Job drawing, mm, ordinate dimensions from the low corner. One solid piece. A direction names the side the tool comes from. Round coordinates to 2 decimals unless told otherwise and drop trailing zeros. Loops run counter-clockwise (first coordinate to the right, second up) from the corner with the lowest first, then second, coordinate; pieces in that order, holes last. Notation, with made-up numbers: M 17,38.25 L 23,38.25 A22 cw 23,63.25 Z; hole C -16,24.5 d8. An arc over 180 degrees is marked long. One line per item, written item: value.
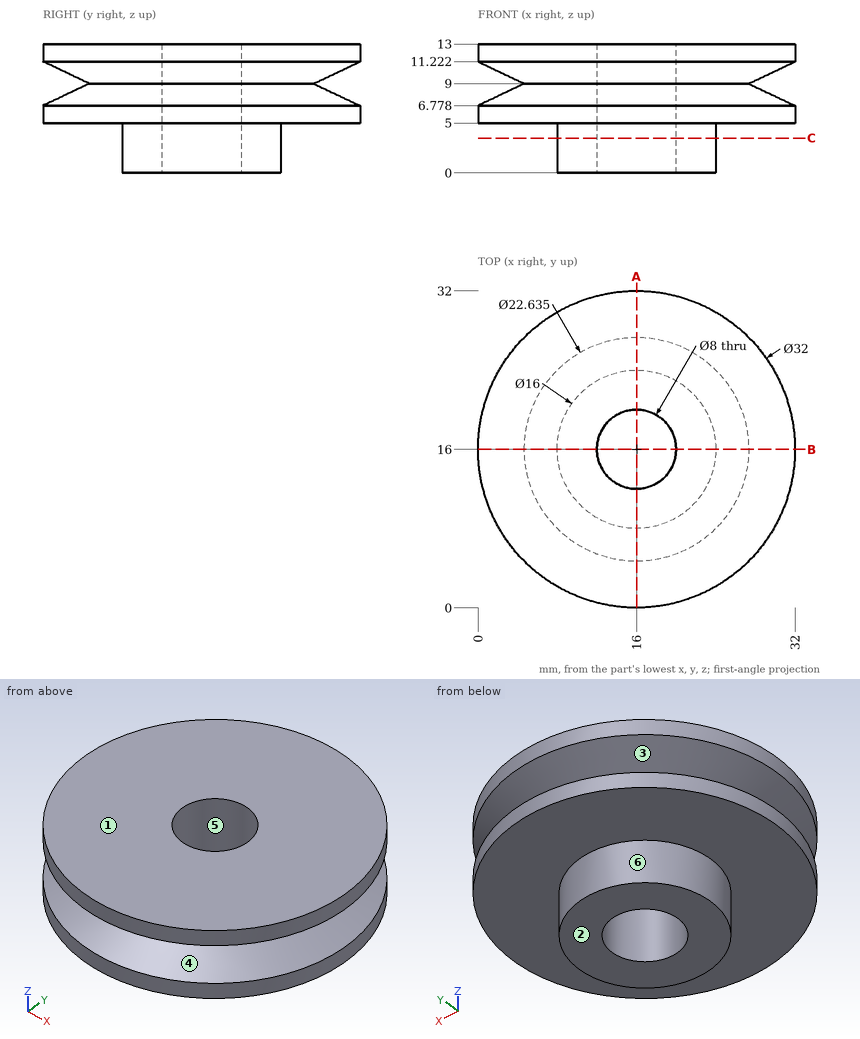
Item 1: Wall check: line 1 along Y through (x, z) = (16, 4); line 2 along Z through (x, y) = (23.5, 10); line 3 along Z through (x, y) = (8.5, 29). Give the ranges that are in metal, low to high.
Check values:
line 1: y = 8 to 12, 20 to 24
line 2: z = 5 to 13
line 3: z = 5 to 7.25, 10.75 to 13
Item 2: Drop flat-ended pins along their axis: P1, Ø2, axis at x = 17, y = 11, coming from the -Z side; P2, Ø1.5, axis at y = 24, z = 4.5, coming from the +X side; P3, Ø1.5, axis at x = 9, z = 3, coming from the -Y side; P4, Ø7, axis at x = 16, y = 16, coming from the -Z side. Give the stop position or say it passes through.
Check values:
P1: stops at z = 0
P2: stops at x = 30.16
P3: stops at y = 11.01
P4: passes through
Item 3: Slice it at A-A, the plane x = 16. Give the cut face in (y, z), and give its area (3 significant figures).
Check values:
outline: M 0,5 L 8,5 L 8,0 L 12,0 L 12,13 L 0,13 L 0,11.22 L 4.68,9 L 0,6.78 Z; M 20,0 L 24,0 L 24,5 L 32,5 L 32,6.78 L 27.32,9 L 32,11.22 L 32,13 L 20,13 Z
area: 211 mm2
Item 4: Which spindle directions (+Z, -Z, +X, -X, +Y, -Y) get a long thin tool onto all of the face, cutting with end or side? Do the marked faces 5 and 6. Say none if no direction does.
Check values:
face 5: +Z, -Z
face 6: -Z
Item 5: Slice it at C-C, the plane z = 3.5. Give the cut face in (x, y), and give its area (3 significant figures).
Check values:
outline: C 16,16 d16; hole C 16,16 d8
area: 151 mm2
Item 6: Pull direction Z, two halves, no side cores. Call the marked faces 1, 2, 3 and 4: pulls with the +Z half, pulls with the -Z half, needs draft (parallel to the pull), parting line crosses it, or undercut.
Check values:
face 1: pulls with the +Z half
face 2: pulls with the -Z half
face 3: undercut
face 4: undercut
